from build123d import *

# Parameters (mm, degrees)
F1_R           = 2.5
F1_R_2         = 17.5
F2_DEPTH       = 5
F3_START       = -3
F1_R_3         = 15
F3_DEPTH       = 2
F4_D           = 5
F4_CSINK_D     = 9
F4_CSINK_ANGLE = 90


with BuildPart() as f2:
    # F1 (on Front) → F2 (new body)
    with BuildSketch(Plane.XZ):
        with BuildLine():
            Line((66.4529909033, 53), (-66.4529909033, 53))
            ThreePointArc((-66.4529909033, 53), (0, -85), (66.4529909033, 53))
        make_face()
        with Locations((0, -75.5)):
            Circle(F1_R, mode=Mode.SUBTRACT)
        with Locations((-58.0947501931, 15)):
            Circle(F1_R, mode=Mode.SUBTRACT)
        Circle(F1_R_2, mode=Mode.SUBTRACT)
        with Locations((58.0947501931, 15)):
            Circle(F1_R, mode=Mode.SUBTRACT)
        with Locations((-58.0947501931, 15)):
            Circle(F1_R)
        with Locations((58.0947501931, 15)):
            Circle(F1_R)
        with Locations((0, -75.5)):
            Circle(F1_R)
    extrude(amount=-F2_DEPTH)

    # F1 (on Front) → F3 (join)
    with BuildSketch(Plane.XZ.offset(F3_START)):
        Circle(F1_R_2)
        Circle(F1_R_3, mode=Mode.SUBTRACT)
    extrude(amount=-F3_DEPTH)

    # F4 (through all)
    with Locations(Plane.XZ):
        with Locations((-58.0947501931, 15), (58.0947501931, 15), (0, -75.5)):
            CounterSinkHole(F4_D / 2, F4_CSINK_D / 2, counter_sink_angle=F4_CSINK_ANGLE)


solid = f2.part
Verification items for the finished model (mm, model axes). A direction names the side the tool comes from. Give positions to 0.01 mm unless a question says otherwise; leave off trailing zeros. Order: outer loops, then holes, each group sorted by start corner. A loop starts at its lowest first (then second) coordinate and runs counter-clockwise, first axis right, second up. Notation, with made-up numbers: M 65.5,-31.5 L 95.5,-31.5 A17 ccw 95.5,-2.5 Z; hole C 20.25,-30 d6. An arc over 180 degrees is marked long. Use one line per item in the form item = value. Start each with the question number.
Q1. Section check A-A (x = 0). Enter the section's corners in (y, z), then the cut area to 3 significant figures.
Q2. Section check D-D (z = -75.5). Enter the section's corners in (x, y), then the cut area to 3 significant figures.
Q3. Go/stop test with flat-tipped pins: pin 1 Ø10 at (x, z) = (-29, 22.5) entering from -Y; pin 2 Ø1.5 at (x, y) = (67.5, 3) entering from +Z; pin 3 Ø2 at (y, z) = (2, 34) entering from -X; pin 4 Ø6 at (x, z) = (-58.09, 15) entering from -Y. Record where each tip stops, or that it passes through.
Q4. Mould release check, pull along X, two halves, no side actions. Record for faces 1 (the cylindrical face through (-55.597, 3.521, 15.11)), 2 (the cylindrical face through (-2.67, 2.46, -84.96)), 3 (the flat face through (1, 2, 53)), 4 (the flat face through (13, 3, 8)): +X half, -X half, draft (parallel to the pull), parting line (faces both ways), or undercut.
Q5. Access from +Z, -Z, +X, -X, +Y, -Y to the whole of each face (thin tool, end or side, straight path). Record for faces 5 (the flat face through (18, 0, -15)), 6 (the cylindrical face through (-13.887, 1.479, -10.648)).
Q6. Scan lines: line 1 along Z through (x, y) = (0, 3.15); line 2 along Z through (x, y) = (1, 3.1); line 3 along Z through (x, y) = (8, 4.2). Record each from-to range of solid material in increasing order. Write a range as [from, to].
Q7. Section check B-B (z = 0). Enter the section's corners in (x, y), then the cut area to 3 significant figures.
Q8. Section check C-C (y = 3.75). Enter the section's corners in (x, z).
Evaluation:
q1.outline = M 0,-85 L 5,-85 L 5,-78 L 2,-78 L 0,-80 Z; M 0,-71 L 2,-73 L 5,-73 L 5,-15 L 3,-15 L 3,-17.5 L 0,-17.5 Z; M 0,17.5 L 3,17.5 L 3,15 L 5,15 L 5,53 L 0,53 Z
q1.area = 496 mm2
q2.outline = M -39.05,0 L -4.5,0 L -2.5,2 L -2.5,5 L -39.05,5 Z; M 2.5,2 L 4.5,0 L 39.05,0 L 39.05,5 L 2.5,5 Z
q2.area = 361 mm2
q3.pin_1 = 0
q3.pin_2 = 52.63
q3.pin_3 = -78.33
q3.pin_4 = 1.5
q4.face_1 = undercut
q4.face_2 = parting line
q4.face_3 = draft
q4.face_4 = undercut
q5.face_5 = +Z, -Z, +X, -X, -Y
q5.face_6 = -Y
q6.line_1 = [-85, -78], [-73, -15], [15, 53]
q6.line_2 = [-84.99, -77.79], [-73.21, -14.97], [14.97, 53]
q6.line_3 = [-84.62, -12.69], [12.69, 53]
q7.outline = M -85,0 L -17.5,0 L -17.5,3 L -15,3 L -15,5 L -85,5 Z; M 15,3 L 17.5,3 L 17.5,0 L 85,0 L 85,5 L 15,5 Z
q7.area = 685 mm2
q8.outline = M -66.45,53 A85 ccw long 66.45,53 Z; hole C -58.09,15 d5; hole C 0,0 d30; hole C 0,-75.5 d5; hole C 58.09,15 d5
